Autodesk Inventor part; units mm, degrees
ref_plane "YZ Plane" through (0, 0, 0) normal (1, 0, 0) x (0, 1, 0)
ref_plane "XZ Plane" through (0, 0, 0) normal (0, 1, 0) x (-1, 0, 0)
ref_plane "XY Plane" through (0, 0, 0) normal (0, 0, 1) x (1, 0, 0)
sketch "Эскиз1" plane through (0, 0, 0) normal (0, 1, 0) x (-1, 0, 0)
  circle A0 centre (-4.9268, 7.9299) radius 1.6
  line L0 (-19.4268, -1.0701) -> (34.5732, -1.0701)
  line L1 (34.5732, -1.0701) -> (34.5732, 36.9299)
  line L2 (34.5732, 36.9299) -> (-19.4268, 36.9299)
  line L3 (-19.4268, 36.9299) -> (-19.4268, -1.0701)
  circle A1 centre (32.1091, 14.2199) radius 1.6
  point P0 (0, 0)
extrude "Выдавливание1" add sketch "Эскиз1" along normal blind 1.7
properties part number "mega_switchboard"
Source: CAD feature listing. Evaluate the final solid. Frame: model axes, mm. Round coordinates to 2 decimals unless told otherwise and drop trailing zeros. Loops run counter-clockwise (first coordinate to the right, second up) from the corner with the lowest first, then second, coordinate; pieces in that order, holes last. Notation, with made-up numbers: (79.5, -40) - (102.5, -40) arc R27 cw to (102.5, -10) - close; hole circle Ø2 at (-31, 56.25). An arc over 180 degrees is marked (long way). Write item = value, one per line. Start each with the question number.
(1) Ray query, line 1 along Z through (x, y) = (6, 0.35); line 2 along X through (y, z) = (1.1, 14.5); line 3 along X through (y, z) = (1.25, 15.5). Return the intervals inside material, ascending. Write a range as from..to.
(2) Section query B-B, the plane x = 4. Output: boundary loops of the cut face in (y, z), plus the area to 3 significant figures.
(3) Section query A-A, the plane z = 8.5. Output: boundary loops of the cut face in (x, y).
(4) Pull-direction query (Z, two-part tool) for faces 1 (the face through (-8, 1, 36.93)), 2 (the face through (-7, 1, -1.07)), 3 (the face through (-7, 1.7, 18)), 4 (the face through (-32.85, 0.84, 15.64)); classes: +Z half, -Z half, draft (parallel to the pull), parting line (faces both ways), or undercut.
Conclusion:
q1.line_1 = -1.07..6.74, 9.12..36.93
q1.line_2 = -34.57..-33.68, -30.53..19.43
q1.line_3 = -34.57..-33.07, -31.15..19.43
q2.outline = (0, -1.07) - (1.7, -1.07) - (1.7, 6.63) - (0, 6.63) - close; (0, 9.23) - (1.7, 9.23) - (1.7, 36.93) - (0, 36.93) - close
q2.area = 60.2 mm2
q3.outline = (-34.57, 0) - (3.43, 0) - (3.43, 1.7) - (-34.57, 1.7) - close; (6.42, 0) - (19.43, 0) - (19.43, 1.7) - (6.42, 1.7) - close
q4.face_1 = +Z half
q4.face_2 = -Z half
q4.face_3 = draft
q4.face_4 = undercut
